Verification items for this drawing (mm, ordinates from the low corner). A direction names the side the tool comes from. Round coordinates to 2 decimals unless told otherwise and drop trailing zeros. Loops run counter-clockwise (first coordinate to the right, second up) from the corner with the lowest first, then second, coordinate; pieces in that order, holes last. Notation, with made-up numbers: M 50,30 L 104,30 A23 ccw 104,62 Z; hole C 59,85 d10. An arc over 180 degrees is marked long. Answer as CSV lines item,"result".
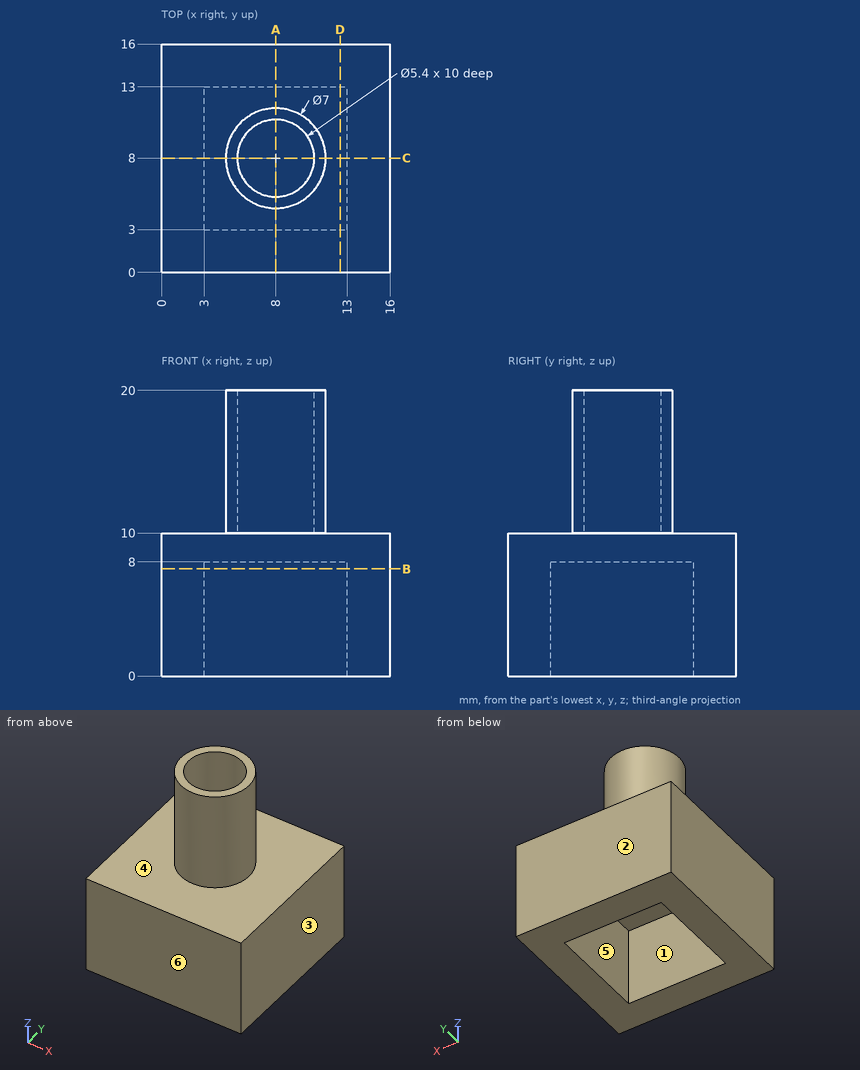
1) Section check B-B (z = 7.5). Record the cut outline in (x, y), plus the area to 3 significant figures.
Here are the results:
outline,"M 0,0 L 16,0 L 16,16 L 0,16 Z; hole M 3,3 L 13,3 L 13,13 L 3,13 Z"
area,"156 mm^2"
2) Draft check along X on the marked faces 1, 2 and 3. Enter one of: +X half, -X half, draft (parallel to the pull), parting line (faces both ways), or undercut.
Here are the results:
face 1,"undercut"
face 2,"draft"
face 3,"+X half"
3) Section check A-A (x = 8). Record the cut outline in (y, z).
Here are the results:
outline,"M 0,0 L 3,0 L 3,8 L 13,8 L 13,0 L 16,0 L 16,10 L 11.5,10 L 11.5,20 L 10.7,20 L 10.7,10 L 5.3,10 L 5.3,20 L 4.5,20 L 4.5,10 L 0,10 Z"
4) Material ranges on probe 1 along Y at (x, z) = (8, 13.75); probe 2 along Y at (x, z) = (5.25, 5), recorded low to high.
Here are the results:
probe 1,"y = 4.5 to 5.3, 10.7 to 11.5"
probe 2,"y = 0 to 3, 13 to 16"
5) Section check D-D (x = 12.5). Record the cut outline in (y, z).
Here are the results:
outline,"M 0,0 L 3,0 L 3,8 L 13,8 L 13,0 L 16,0 L 16,10 L 0,10 Z"
6) Go/stop test with a flat-tipped pin: pin 1 (2.5 mm diameter, centred on x = 7.5, y = 9, fed in from +Z). Record where the tip stops, or that it passes through.
Here are the results:
pin 1,"stops at z = 10"
7) Set-up check for the marked faces 4, 5 and 6: record each of +Z, -Z, +X, -X, +Y, -Y from which the full face is reachable in a straight line by a thin tool's end or side.
Here are the results:
face 4,"+Z"
face 5,"-Z"
face 6,"+Z, -Z, +X, -X, -Y"
